```python
from build123d import *

# Parameters (mm, degrees)
BOSS_EXTRUDE1_DEPTH = 4
SKETCH2_R           = 1.5
CUT_EXTRUDE1_DEPTH  = 4
SKETCH6_R           = 1.05
CUT_EXTRUDE2_DEPTH  = 4
CUT_EXTRUDE3_DEPTH  = 40.517337967


with BuildPart() as part:
    # Sketch1 → Boss-Extrude1 (new body)
    with BuildSketch(Plane(origin=(0, 0, 0), x_dir=(1, 0, 0), z_dir=(0, 1, 0))):
        with BuildLine():
            Line((35, -4.1), (-35, -4.1))
            ThreePointArc((-35, -4.1), (-39.1, 0), (-35, 4.1))
            Line((-35, 4.1), (35, 4.1))
            ThreePointArc((35, 4.1), (39.1, 0), (35, -4.1))
        make_face()
    extrude(amount=-BOSS_EXTRUDE1_DEPTH)

    # Sketch2 → Cut-Extrude1 (cut)
    with BuildSketch(Plane(origin=(0, 0, 0), x_dir=(1, 0, 0), z_dir=(0, 1, 0))):
        with Locations(Location((0, 0, 0), (0, 0, 270))):
            Circle(SKETCH2_R)
    extrude(amount=-CUT_EXTRUDE1_DEPTH, mode=Mode.SUBTRACT)

    # Sketch6 → Cut-Extrude2 (cut)
    with BuildSketch(Plane(origin=(0, 0, 0), x_dir=(1, 0, 0), z_dir=(0, 1, 0))):
        with Locations(Location((-35, 0, 0), (0, 0, 270))):
            Circle(SKETCH6_R)
    cut_extrude2 = extrude(amount=-CUT_EXTRUDE2_DEPTH, mode=Mode.SUBTRACT)

    # Sketch7 → Cut-Extrude3 (cut, through all)
    with BuildSketch(Plane(origin=(0, 0, 0), x_dir=(1, 0, 0), z_dir=(0, 1, 0))):
        with BuildLine():
            Line((-29.375, 1.625), (-5.625, 1.625))
            ThreePointArc((-5.625, 1.625), (-4, 0), (-5.625, -1.625))
            Line((-5.625, -1.625), (-29.375, -1.625))
            ThreePointArc((-29.375, -1.625), (-31, 0), (-29.375, 1.625))
        make_face()
    cut_extrude3 = extrude(amount=-CUT_EXTRUDE3_DEPTH, mode=Mode.SUBTRACT)

    # Mirror1: Cut-Extrude2, Cut-Extrude3 across plane
    add(cut_extrude2.mirror(Plane(origin=(0, 0, 0), x_dir=(0, 0, 1), z_dir=(1, 0, 0))), mode=Mode.SUBTRACT)
    add(cut_extrude3.mirror(Plane(origin=(0, 0, 0), x_dir=(0, 0, 1), z_dir=(1, 0, 0))), mode=Mode.SUBTRACT)


solid = part.part
```
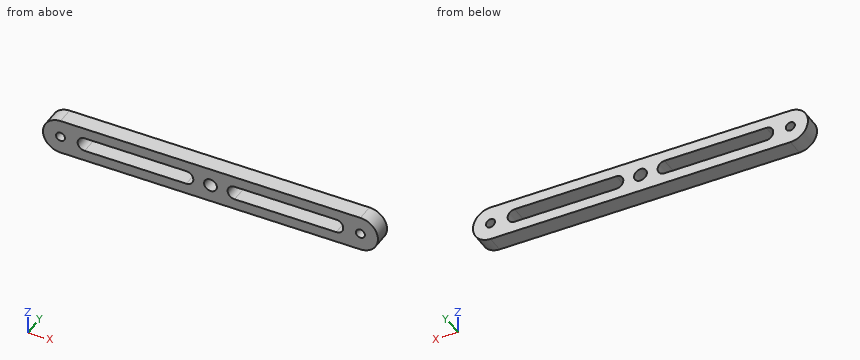
The model under review builds one solid part; all positions refer to its coordinate system, in mm. Give positions to 0.01 mm unless a question says otherwise; leave off trailing zeros. Loops run counter-clockwise (first coordinate to the right, second up) from the corner with the lowest first, then second, coordinate; pieces in that order, holes last. Notation, with made-up numbers: (-30.5, 42.5) - (-2.5, 42.5) arc R12 cw to (-2.5, 57.5) - close; hole circle Ø10 at (18, 29.5). An arc over 180 degrees is marked (long way). Answer as a JSON object with one key per item and string values.
Q1. To check wall thickness, follow line 1 along X through (y, z) = (-2, 0); line 2 along Z through (x, y) = (-28.5, -1.3) (3 decimals); line 3 along X through (y, z) = (-2, -1.25). State the ranges of each line that lie inside material, in increasing order.
Worked out:
{"line 1": "x = -39.1 to -36.05, -33.95 to -31, -4 to -1.5, 1.5 to 4, 31 to 33.95, 36.05 to 39.1", "line 2": "z = -4.1 to -1.625, 1.625 to 4.1", "line 3": "x = -38.9 to -30.41, -4.59 to -0.83, 0.83 to 4.59, 30.41 to 38.9"}
Q2. Add section C-C on x = 0. State the section outline as (y, z) points, plus the area to 3 significant figures.
Worked out:
{"outline": "(-4, -4.1) - (0, -4.1) - (0, -1.5) - (-4, -1.5) - close; (-4, 1.5) - (0, 1.5) - (0, 4.1) - (-4, 4.1) - close", "area": "20.8 mm^2"}
Q3. Add section A-A on z = 0. State the section outline as (x, y) points.
Worked out:
{"outline": "(-39.1, -4) - (-36.05, -4) - (-36.05, 0) - (-39.1, 0) - close; (-33.95, -4) - (-31, -4) - (-31, 0) - (-33.95, 0) - close; (-4, -4) - (-1.5, -4) - (-1.5, 0) - (-4, 0) - close; (1.5, -4) - (4, -4) - (4, 0) - (1.5, 0) - close; (31, -4) - (33.95, -4) - (33.95, 0) - (31, 0) - close; (36.05, -4) - (39.1, -4) - (39.1, 0) - (36.05, 0) - close"}
Q4. Add section B-B on y = -3.25. State the section outline as (x, z) points (3 decimals), plus the area to 3 significant figures.
Worked out:
{"outline": "(-35, -4.1) - (35, -4.1) arc R4.1 ccw to (35, 4.1) - (-35, 4.1) arc R4.1 ccw to start; hole circle Ø2.1 at (-35, 0); hole (-29.375, -1.625) - (-5.625, -1.625) arc R1.625 ccw to (-5.625, 1.625) - (-29.375, 1.625) arc R1.625 ccw to start; hole circle Ø3 at (0, 0); hole (5.625, -1.625) - (29.375, -1.625) arc R1.625 ccw to (29.375, 1.625) - (5.625, 1.625) arc R1.625 ccw to start; hole circle Ø2.1 at (35, 0)", "area": "442 mm^2"}
Q5. Insertion check: pin 1 (1.5 mm diameter, centred on y = -1.5, z = -2.5, fed in from -X). The pin has a flat end and moves straight along its axis. Give the tip position at first contact, or say it passes through.
Worked out:
{"pin 1": "stops at x = -38.71"}
